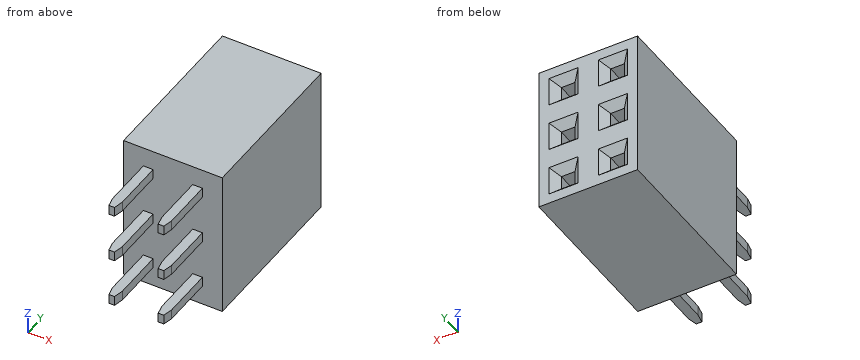
```python
from build123d import *
from OCP.BRepFilletAPI import BRepFilletAPI_MakeChamfer

# Parameters (mm, degrees)
SKETCH_1_W                          = 2.54
SKETCH_1_H                          = 2.54
EXTRUDE_1_DEPTH                     = 8.51
SKETCH_4_W                          = 0.7
SKETCH_4_H                          = 0.7
CUT_EXTRUDE_1_DEPTH                 = 8.21
CHAMFER_3_SIZE                      = 0.4
SKETCH_2_W                          = 0.5
SKETCH_2_H                          = 0.5
EXTRUDE_2_DEPTH                     = 3.15
CHAMFER_2_SIZE                      = 0.5
CHAMFER_2_SIZE2                     = 0.106278281
PATTERN_LINEAR_1_COUNT              = 3
PATTERN_LINEAR_1_PITCH              = 2.54
PATTERN_LINEAR_1_COUNT_DIR2         = 2
PATTERN_LINEAR_1_PITCH_DIR2         = 2.54
CHAMFER_3_OF_PATTERN_LINEAR_1_SIZE  = 0.4
CHAMFER_2_OF_PATTERN_LINEAR_1_SIZE  = 0.5
CHAMFER_2_OF_PATTERN_LINEAR_1_SIZE2 = 0.106278281


with BuildPart() as part:
    # Эскиз1 → Бобышка-Вытянуть1 (new body)
    with BuildSketch(Plane(origin=(0, 0, 0), x_dir=(-1, 0, 0), z_dir=(0, 1, 0))):
        Rectangle(SKETCH_1_W, SKETCH_1_H)
    extrude_1 = extrude(amount=EXTRUDE_1_DEPTH)

    # Эскиз4 → Вырез-Вытянуть1 (cut)
    with BuildSketch(Plane(origin=(0, 8.51, 0), x_dir=(1, 0, 0), z_dir=(0, 1, 0))):
        Rectangle(SKETCH_4_W, SKETCH_4_H)
    cut_extrude_1 = extrude(amount=-CUT_EXTRUDE_1_DEPTH, mode=Mode.SUBTRACT)

    # Фаска3
    chamfer_3_edges = [part.edges().sort_by_distance(p)[0] for p in [
        (-0.35, 8.51, 0),
        (0, 8.51, 0.35),
        (0.35, 8.51, 0),
        (0, 8.51, -0.35),
    ]]
    chamfer(chamfer_3_edges, length=CHAMFER_3_SIZE)

    # Эскиз2 → Бобышка-Вытянуть2 (add)
    with BuildSketch(Plane(origin=(0, 0, 0), x_dir=(-1, 0, 0), z_dir=(0, 1, 0))):
        Rectangle(SKETCH_2_W, SKETCH_2_H)
    extrude_2 = extrude(amount=-EXTRUDE_2_DEPTH)

    # Фаска2: one chamfer whose edges measure the first distance from different faces: ONE call of the kernel's chamfer builder (chamfer() names one face for all edges)
    chamfer_2_edges_1 = [part.edges().sort_by_distance(p)[0] for p in [
        (-0.25, -3.15, 0),
    ]]
    chamfer_2_side_1 = [part.faces().sort_by_distance(p)[0] for p in [
        (-0.25, -1.575, 0),
    ]]
    chamfer_2_edges_2 = [part.edges().sort_by_distance(p)[0] for p in [
        (0.25, -3.15, 0),
    ]]
    chamfer_2_side_2 = [part.faces().sort_by_distance(p)[0] for p in [
        (0.25, -1.575, 0),
    ]]
    chamfer_2 = BRepFilletAPI_MakeChamfer(part.part.solid().wrapped)
    for e in chamfer_2_edges_1:
        chamfer_2.Add(CHAMFER_2_SIZE, CHAMFER_2_SIZE2, e.wrapped, chamfer_2_side_1[0].wrapped)  # the first distance lies on this face
    for e in chamfer_2_edges_2:
        chamfer_2.Add(CHAMFER_2_SIZE, CHAMFER_2_SIZE2, e.wrapped, chamfer_2_side_2[0].wrapped)  # the first distance lies on this face
    add(Compound.cast(chamfer_2.Shape()), mode=Mode.REPLACE)

    # Линейный массив1: Бобышка-Вытянуть1, Вырез-Вытянуть1, Extrude 2 3 × 2
    with Locations(*[(-j * PATTERN_LINEAR_1_PITCH_DIR2, 0, -i * PATTERN_LINEAR_1_PITCH) for i in range(PATTERN_LINEAR_1_COUNT) for j in range(PATTERN_LINEAR_1_COUNT_DIR2) if (i, j) != (0, 0)]):
        add(extrude_1)
        add(cut_extrude_1, mode=Mode.SUBTRACT)
        add(extrude_2)

    # Фаска3 of Линейный массив1
    chamfer_3_of_pattern_linear_1_edges = [part.edges().sort_by_distance(p)[0] for p in [
        (-2.89, 8.51, 0),
        (-2.54, 8.51, 0.35),
        (-2.19, 8.51, 0),
        (-2.54, 8.51, -0.35),
        (-0.35, 8.51, -2.54),
        (0, 8.51, -2.19),
        (0.35, 8.51, -2.54),
        (0, 8.51, -2.89),
        (-2.89, 8.51, -2.54),
        (-2.54, 8.51, -2.19),
        (-2.19, 8.51, -2.54),
        (-2.54, 8.51, -2.89),
        (-0.35, 8.51, -5.08),
        (0, 8.51, -4.73),
        (0.35, 8.51, -5.08),
        (0, 8.51, -5.43),
        (-2.89, 8.51, -5.08),
        (-2.54, 8.51, -4.73),
        (-2.19, 8.51, -5.08),
        (-2.54, 8.51, -5.43),
    ]]
    chamfer(chamfer_3_of_pattern_linear_1_edges, length=CHAMFER_3_OF_PATTERN_LINEAR_1_SIZE)

    # Фаска2 of Линейный массив1: one chamfer whose edges measure the first distance from different faces: ONE call of the kernel's chamfer builder (chamfer() names one face for all edges)
    chamfer_2_of_pattern_linear_1_edges_1 = [part.edges().sort_by_distance(p)[0] for p in [
        (-2.79, -3.15, 0),
    ]]
    chamfer_2_of_pattern_linear_1_side_1 = [part.faces().sort_by_distance(p)[0] for p in [
        (-2.79, -1.575, 0),
    ]]
    chamfer_2_of_pattern_linear_1_edges_2 = [part.edges().sort_by_distance(p)[0] for p in [
        (-2.29, -3.15, 0),
    ]]
    chamfer_2_of_pattern_linear_1_side_2 = [part.faces().sort_by_distance(p)[0] for p in [
        (-2.29, -1.575, 0),
    ]]
    chamfer_2_of_pattern_linear_1_edges_3 = [part.edges().sort_by_distance(p)[0] for p in [
        (-0.25, -3.15, -2.54),
    ]]
    chamfer_2_of_pattern_linear_1_side_3 = [part.faces().sort_by_distance(p)[0] for p in [
        (-0.25, -1.575, -2.54),
    ]]
    chamfer_2_of_pattern_linear_1_edges_4 = [part.edges().sort_by_distance(p)[0] for p in [
        (0.25, -3.15, -2.54),
    ]]
    chamfer_2_of_pattern_linear_1_side_4 = [part.faces().sort_by_distance(p)[0] for p in [
        (0.25, -1.575, -2.54),
    ]]
    chamfer_2_of_pattern_linear_1_edges_5 = [part.edges().sort_by_distance(p)[0] for p in [
        (-2.79, -3.15, -2.54),
    ]]
    chamfer_2_of_pattern_linear_1_side_5 = [part.faces().sort_by_distance(p)[0] for p in [
        (-2.79, -1.575, -2.54),
    ]]
    chamfer_2_of_pattern_linear_1_edges_6 = [part.edges().sort_by_distance(p)[0] for p in [
        (-2.29, -3.15, -2.54),
    ]]
    chamfer_2_of_pattern_linear_1_side_6 = [part.faces().sort_by_distance(p)[0] for p in [
        (-2.29, -1.575, -2.54),
    ]]
    chamfer_2_of_pattern_linear_1_edges_7 = [part.edges().sort_by_distance(p)[0] for p in [
        (-0.25, -3.15, -5.08),
    ]]
    chamfer_2_of_pattern_linear_1_side_7 = [part.faces().sort_by_distance(p)[0] for p in [
        (-0.25, -1.575, -5.08),
    ]]
    chamfer_2_of_pattern_linear_1_edges_8 = [part.edges().sort_by_distance(p)[0] for p in [
        (0.25, -3.15, -5.08),
    ]]
    chamfer_2_of_pattern_linear_1_side_8 = [part.faces().sort_by_distance(p)[0] for p in [
        (0.25, -1.575, -5.08),
    ]]
    chamfer_2_of_pattern_linear_1_edges_9 = [part.edges().sort_by_distance(p)[0] for p in [
        (-2.79, -3.15, -5.08),
    ]]
    chamfer_2_of_pattern_linear_1_side_9 = [part.faces().sort_by_distance(p)[0] for p in [
        (-2.79, -1.575, -5.08),
    ]]
    chamfer_2_of_pattern_linear_1_edges_10 = [part.edges().sort_by_distance(p)[0] for p in [
        (-2.29, -3.15, -5.08),
    ]]
    chamfer_2_of_pattern_linear_1_side_10 = [part.faces().sort_by_distance(p)[0] for p in [
        (-2.29, -1.575, -5.08),
    ]]
    chamfer_2_of_pattern_linear_1 = BRepFilletAPI_MakeChamfer(part.part.solid().wrapped)
    for e in chamfer_2_of_pattern_linear_1_edges_1:
        chamfer_2_of_pattern_linear_1.Add(CHAMFER_2_OF_PATTERN_LINEAR_1_SIZE, CHAMFER_2_OF_PATTERN_LINEAR_1_SIZE2, e.wrapped, chamfer_2_of_pattern_linear_1_side_1[0].wrapped)  # the first distance lies on this face
    for e in chamfer_2_of_pattern_linear_1_edges_2:
        chamfer_2_of_pattern_linear_1.Add(CHAMFER_2_OF_PATTERN_LINEAR_1_SIZE, CHAMFER_2_OF_PATTERN_LINEAR_1_SIZE2, e.wrapped, chamfer_2_of_pattern_linear_1_side_2[0].wrapped)  # the first distance lies on this face
    for e in chamfer_2_of_pattern_linear_1_edges_3:
        chamfer_2_of_pattern_linear_1.Add(CHAMFER_2_OF_PATTERN_LINEAR_1_SIZE, CHAMFER_2_OF_PATTERN_LINEAR_1_SIZE2, e.wrapped, chamfer_2_of_pattern_linear_1_side_3[0].wrapped)  # the first distance lies on this face
    for e in chamfer_2_of_pattern_linear_1_edges_4:
        chamfer_2_of_pattern_linear_1.Add(CHAMFER_2_OF_PATTERN_LINEAR_1_SIZE, CHAMFER_2_OF_PATTERN_LINEAR_1_SIZE2, e.wrapped, chamfer_2_of_pattern_linear_1_side_4[0].wrapped)  # the first distance lies on this face
    for e in chamfer_2_of_pattern_linear_1_edges_5:
        chamfer_2_of_pattern_linear_1.Add(CHAMFER_2_OF_PATTERN_LINEAR_1_SIZE, CHAMFER_2_OF_PATTERN_LINEAR_1_SIZE2, e.wrapped, chamfer_2_of_pattern_linear_1_side_5[0].wrapped)  # the first distance lies on this face
    for e in chamfer_2_of_pattern_linear_1_edges_6:
        chamfer_2_of_pattern_linear_1.Add(CHAMFER_2_OF_PATTERN_LINEAR_1_SIZE, CHAMFER_2_OF_PATTERN_LINEAR_1_SIZE2, e.wrapped, chamfer_2_of_pattern_linear_1_side_6[0].wrapped)  # the first distance lies on this face
    for e in chamfer_2_of_pattern_linear_1_edges_7:
        chamfer_2_of_pattern_linear_1.Add(CHAMFER_2_OF_PATTERN_LINEAR_1_SIZE, CHAMFER_2_OF_PATTERN_LINEAR_1_SIZE2, e.wrapped, chamfer_2_of_pattern_linear_1_side_7[0].wrapped)  # the first distance lies on this face
    for e in chamfer_2_of_pattern_linear_1_edges_8:
        chamfer_2_of_pattern_linear_1.Add(CHAMFER_2_OF_PATTERN_LINEAR_1_SIZE, CHAMFER_2_OF_PATTERN_LINEAR_1_SIZE2, e.wrapped, chamfer_2_of_pattern_linear_1_side_8[0].wrapped)  # the first distance lies on this face
    for e in chamfer_2_of_pattern_linear_1_edges_9:
        chamfer_2_of_pattern_linear_1.Add(CHAMFER_2_OF_PATTERN_LINEAR_1_SIZE, CHAMFER_2_OF_PATTERN_LINEAR_1_SIZE2, e.wrapped, chamfer_2_of_pattern_linear_1_side_9[0].wrapped)  # the first distance lies on this face
    for e in chamfer_2_of_pattern_linear_1_edges_10:
        chamfer_2_of_pattern_linear_1.Add(CHAMFER_2_OF_PATTERN_LINEAR_1_SIZE, CHAMFER_2_OF_PATTERN_LINEAR_1_SIZE2, e.wrapped, chamfer_2_of_pattern_linear_1_side_10[0].wrapped)  # the first distance lies on this face
    add(Compound.cast(chamfer_2_of_pattern_linear_1.Shape()), mode=Mode.REPLACE)


solid = part.part
```
Design review of the part built by this model. Coordinates are the model's own, in mm. Round coordinates to 2 decimals unless told otherwise and drop trailing zeros. Order: outer loops, then holes, each group sorted by start corner. A loop starts at its lowest first (then second) coordinate and runs counter-clockwise, first axis right, second up. Notation, with made-up numbers: (50, 31) - (65, 31) arc R31 ccw to (65, 70) - close; hole circle Ø6 at (62.25, 1.5). An arc over 180 degrees is marked (long way). One line per question, with ' | ' between items.
Item 1: For P1, Ø0.6, axis at y = -1, z = -5, coming from the +X side; P2, Ø1.5, axis at x = -2, y = -1.5, coming from the -Z side, all flat-tipped, find the tip position at first contact; note any pin that passes through.
Checks:
P1: x = 0.25 | P2: z = -5.33
Item 2: Wall thickness on line 1 (Z direction, x = 0.1, y = 3.25); line 2 (X direction, y = 1.75, z = -5): over which ranges is each line inside the solid? List them lowest first. Write a range as [from, to].
Checks:
line 1: [-6.35, -5.43], [-4.73, -2.89], [-2.19, -0.35], [0.35, 1.27] | line 2: [-3.81, -2.89], [-2.19, -0.35], [0.35, 1.27]
Item 3: Take a section at A-A, the plane y = 2. Write out the cut boundary in (x, z), then the cut area to 3 significant figures.
Checks:
outline: (-3.81, -6.35) - (1.27, -6.35) - (1.27, 1.27) - (-3.81, 1.27) - close; hole (-2.89, -5.43) - (-2.19, -5.43) - (-2.19, -4.73) - (-2.89, -4.73) - close; hole (-2.89, -2.89) - (-2.19, -2.89) - (-2.19, -2.19) - (-2.89, -2.19) - close; hole (-2.89, -0.35) - (-2.19, -0.35) - (-2.19, 0.35) - (-2.89, 0.35) - close; hole (-0.35, -5.43) - (0.35, -5.43) - (0.35, -4.73) - (-0.35, -4.73) - close; hole (-0.35, -2.89) - (0.35, -2.89) - (0.35, -2.19) - (-0.35, -2.19) - close; hole (-0.35, -0.35) - (0.35, -0.35) - (0.35, 0.35) - (-0.35, 0.35) - close | area: 35.8 mm²
Item 4: Take a section at D-D, the plane z = 0.5. Write out the cut boundary in (x, y), then the cut area to 3 significant figures.
Checks:
outline: (-3.81, 0) - (1.27, 0) - (1.27, 8.51) - (0.75, 8.51) - (0.5, 8.26) - (-0.5, 8.26) - (-0.75, 8.51) - (-1.79, 8.51) - (-2.04, 8.26) - (-3.04, 8.26) - (-3.29, 8.51) - (-3.81, 8.51) - close | area: 42.6 mm²
Item 5: Take a section at C-C, the plane x = -3.05. Write out the cut boundary in (y, z), then the cut area to 3 significant figures.
Checks:
outline: (0, -6.35) - (8.51, -6.35) - (8.51, -5.83) - (8.27, -5.59) - (8.27, -4.57) - (8.51, -4.33) - (8.51, -3.29) - (8.27, -3.05) - (8.27, -2.03) - (8.51, -1.79) - (8.51, -0.75) - (8.27, -0.51) - (8.27, 0.51) - (8.51, 0.75) - (8.51, 1.27) - (0, 1.27) - close | area: 63.9 mm²
Item 6: Take a section at B-B, the plane z = -4.5. Write out the cut boundary in (x, y).
Checks:
outline: (-3.81, 0) - (1.27, 0) - (1.27, 8.51) - (0.75, 8.51) - (0.58, 8.34) - (-0.58, 8.34) - (-0.75, 8.51) - (-1.79, 8.51) - (-1.96, 8.34) - (-3.12, 8.34) - (-3.29, 8.51) - (-3.81, 8.51) - close
